Verification items for the finished model (mm, model axes). A direction names the side the tool comes from. Give positions to 0.01 mm unless a question says otherwise; leave off trailing zeros. Loops run counter-clockwise (first coordinate to the right, second up) from the corner with the lowest first, then second, coordinate; pieces in that order, holes last. Notation, with made-up numbers: M 11.25,14.25 L 33.25,14.25 A27 ccw 33.25,53.25 Z; hole C 20.25,50 d2. An arc over 180 degrees is marked long. Put each result on its own line as item: value. Start each with the question number.
from build123d import *

# Parameters (mm, degrees)
F0_R         = 0.5
F1_DEPTH     = 9
F2_T1_DEPTH  = 1.9538472674
F2_T3_DEPTH  = 1.9538472674
F2_T5_DEPTH  = 1.9538472674
F2_T7_DEPTH  = 1.9538472674
F2_T9_DEPTH  = 1.9538472674
F2_T11_DEPTH = 1.9538472674
F2_T13_DEPTH = 1.9538472674
F3_DEPTH     = 0.5


# Not quite as in the source:
# - a fillet or chamfer that OpenCascade refuses, or shapes differently, is made with other operations: its cross-section is extruded or revolved along the edge and cut away or added


with BuildPart() as f1:
    # F0 (on Front) → F1 (new body)
    with BuildSketch(Plane.XZ):
        Polygon((1.2, 0.1455782856), (0.7455887445, 0.9514675304), (-0.1455782856, 1.2), (-0.9514675304, 0.7455887445), (-1.2, -0.1455782856), (-0.7455887445, -0.9514675304), (0.1455782856, -1.2), (0.9514675304, -0.7455887445), align=None)
        Circle(F0_R, mode=Mode.SUBTRACT)
    extrude(amount=F1_DEPTH)

    # F2: chamfer of 0.2 on 8 edges, made by hand

    # F2_s2 → F2_t1 (cut)
    with BuildSketch(Plane(origin=(0.8509666159, 0, 0.4798287244), x_dir=(0, 1, 0), z_dir=(-0.871067693, 0, -0.4911629813))):
        Polygon((-8.8, -1.1167838964), (-9, -0.9167838964), (-9, -1.1167838964), align=None)
    extrude(amount=F2_T1_DEPTH, mode=Mode.SUBTRACT)

    # F2_s4 → F2_t3 (cut)
    with BuildSketch(Plane(origin=(0.2624341198, 0, 0.9410144095), x_dir=(0, 1, 0), z_dir=(-0.2686331979, 0, -0.9632425473))):
        Polygon((-8.8, -1.1167838964), (-9, -0.9167838964), (-9, -1.1167838964), align=None)
    extrude(amount=F2_T3_DEPTH, mode=Mode.SUBTRACT)

    # F2_s6 → F2_t5 (cut)
    with BuildSketch(Plane(origin=(-0.4798287244, 0, 0.8509666159), x_dir=(0, 1, 0), z_dir=(0.4911629813, 0, -0.871067693))):
        Polygon((-8.8, -1.1167838964), (-9, -0.9167838964), (-9, -1.1167838964), align=None)
    extrude(amount=F2_T5_DEPTH, mode=Mode.SUBTRACT)

    # F2_s8 → F2_t7 (cut)
    with BuildSketch(Plane(origin=(-0.8509666159, 0, -0.4798287244), x_dir=(0, 1, 0), z_dir=(0.871067693, 0, 0.4911629813))):
        Polygon((-8.8, -1.1167838964), (-9, -0.9167838964), (-9, -1.1167838964), align=None)
    extrude(amount=F2_T7_DEPTH, mode=Mode.SUBTRACT)

    # F2_s10 → F2_t9 (cut)
    with BuildSketch(Plane(origin=(-0.2624341198, 0, -0.9410144095), x_dir=(0, 1, 0), z_dir=(0.2686331979, 0, 0.9632425473))):
        Polygon((-8.8, -1.1167838964), (-9, -0.9167838964), (-9, -1.1167838964), align=None)
    extrude(amount=F2_T9_DEPTH, mode=Mode.SUBTRACT)

    # F2_s12 → F2_t11 (cut)
    with BuildSketch(Plane(origin=(0.4798287244, 0, -0.8509666159), x_dir=(0, 1, 0), z_dir=(-0.4911629813, 0, 0.871067693))):
        Polygon((-8.8, -1.1167838964), (-9, -0.9167838964), (-9, -1.1167838964), align=None)
    extrude(amount=F2_T11_DEPTH, mode=Mode.SUBTRACT)

    # F2_s14 → F2_t13 (cut)
    with BuildSketch(Plane(origin=(0.9410144095, 0, -0.2624341198), x_dir=(0, 1, 0), z_dir=(-0.9632425473, 0, 0.2686331979))):
        Polygon((-8.8, -1.1167838964), (-9, -0.9167838964), (-9, -1.1167838964), align=None)
    extrude(amount=F2_T13_DEPTH, mode=Mode.SUBTRACT)

    # F0 (on Front) → F3 (join)
    with BuildSketch(Plane.XZ):
        with BuildLine():
            Line((-0.1455782856, 1.2), (0.7455887445, 0.9514675304))
            Line((0.7455887445, 0.9514675304), (1.2, 0.1455782856))
            Line((1.2, 0.1455782856), (0.9514675304, -0.7455887445))
            Line((0.9514675304, -0.7455887445), (0.1455782856, -1.2))
            Line((0.1455782856, -1.2), (0.6645818987, -1.3447419455))
            ThreePointArc((0.6645818987, -1.3447419455), (1.2741414458, -0.7915576896), (1.5, 0))
            ThreePointArc((1.5, 0), (-0.4201853542, 1.4399459254), (-1.2645923575, -0.8067255849))
            Line((-1.2645923575, -0.8067255849), (-0.7455887445, -0.9514675304))
            Line((-0.7455887445, -0.9514675304), (-1.2, -0.1455782856))
            Line((-1.2, -0.1455782856), (-0.9514675304, 0.7455887445))
            Line((-0.9514675304, 0.7455887445), (-0.1455782856, 1.2))
        make_face()
        Polygon((1.2, 0.1455782856), (0.7455887445, 0.9514675304), (-0.1455782856, 1.2), (-0.9514675304, 0.7455887445), (-1.2, -0.1455782856), (-0.7455887445, -0.9514675304), (0.1455782856, -1.2), (0.9514675304, -0.7455887445), align=None)
        Circle(F0_R, mode=Mode.SUBTRACT)
        Circle(F0_R)
    extrude(amount=-F3_DEPTH)


solid = f1.part
Q1. Cross-section at D-D, the plane z = 0.25. Record the boundary of the cut face in (x, y), then the cut area to 3 significant figures.
Q2. Scan lines: L1, parallel to Z at x = 0, y = -5.5; L2, parallel to Y at x = 1.2, z = 0.8; L3, parallel to X at y = -3, z = 0.05. Record each from-to range of solid material in increasing order.
Q3. Go/stop test with flat-tipped pins: pin 1 (1 mm diameter, centred on y = -6.5, z = -1, fed in from -X); pin 2 (1 mm diameter, centred on x = 1, y = -6.5, fed in from +Z). Record where each tip stops, or that it passes through.
Q4. Release check for a two-part mould opening along Z. For faces 1 (the face through (0.5, -4.3, -1)), 2 (the face through (0, 0.5, 0)), 3 (the face through (-0.108, -4.437, -0.488)), 4 (the face through (-0.5, -4.3, 1)) record: pulls with the +Z half, pulls with the -Z half, needs draft (parallel to the pull), parting line crosses it, or undercut.
Q5. Set-up check for faces 5 (the face through (-1, -4.3, -0.5)), 6 (the face through (1, -4.3, 0.5)), 7 (the face through (-1.074, -4.338, 0.306)): record each of +Z, -Z, +X, -X, +Y, -Y from which the full face is reachable in a straight line by a thin tool's end or side.
Q6. Cross-section at A-A, the plane y = -4.5. Record the boundary of the cut face in (x, z), then the cut area to 3 significant figures.
Q7. Cross-section at B-B, the plane z = -0.3. Record the boundary of the cut face in (x, y), then the cut area to 3 significant figures.
Q8. Cross-section at C-C, the plane x = 1.1. Record the boundary of the cut face in (y, z).
Ans:
1. outline: M -1.48,0 L -1.09,0 L -1.09,-8.8 L -0.88,-9 L -0.43,-9 L -0.43,0 L 0.43,0 L 0.43,-9 L 0.91,-9 L 1.14,-8.8 L 1.14,0 L 1.48,0 L 1.48,0.5 L -1.48,0.5 Z
1. area: 13.7 mm^2
2. L1: z = -1.16 to -0.5, 0.5 to 1.16
2. L2: y = 0 to 0.5
2. L3: x = -1.15 to -0.5, 0.5 to 1.17
3. pin 1: stops at x = -1
3. pin 2: stops at z = 1.02
4. face 1: pulls with the -Z half
4. face 2: needs draft
4. face 3: undercut
4. face 4: pulls with the +Z half
5. face 5: -Z, -X, -Y
5. face 6: +Z, +X, -Y
5. face 7: +Z, -X, -Y
6. outline: M -1.2,-0.15 L -0.75,-0.95 L 0.15,-1.2 L 0.95,-0.75 L 1.2,0.15 L 0.75,0.95 L -0.15,1.2 L -0.95,0.75 Z; hole C 0,0 d1
6. area: 3.35 mm^2
7. outline: M -1.47,0 L -1.11,0 L -1.11,-8.8 L -0.88,-9 L -0.4,-9 L -0.4,0 L 0.4,0 L 0.4,-9 L 0.87,-9 L 1.08,-8.8 L 1.08,0 L 1.47,0 L 1.47,0.5 L -1.47,0.5 Z
7. area: 13.9 mm^2
8. outline: M -8.89,0.13 L -8.8,-0.21 L 0,-0.21 L 0,-1.02 L 0.5,-1.02 L 0.5,1.02 L 0,1.02 L 0,0.32 L -8.8,0.32 Z
